```python
from build123d import *

# Parameters (mm, degrees)
BOSS_EXTRUDE1_DEPTH = 30
SKETCH2_W           = 3
SKETCH2_H           = 22
CUT_EXTRUDE1_DEPTH  = 75.999903187
FILLET2_R           = 10
SKETCH5_R           = 2
CUT_EXTRUDE2_DEPTH  = 0.5
SKETCH8_R           = 1
CUT_EXTRUDE3_DEPTH  = 75.983234646
FILLET3_R           = 1
FILLET4_R           = 0.75


with BuildPart() as part:
    # Sketch1 → Boss-Extrude1 (new body)
    with BuildSketch(Plane(origin=(0, 0, 0), x_dir=(1, 0, 0), z_dir=(0, 1, 0))):
        with BuildLine():
            Line((2.436698586, 0.75), (68.683498586, 0.75))
            Line((68.683498586, 0.75), (68.683498586, -0.75))
            Line((68.683498586, -0.75), (2.436698586, -0.75))
            ThreePointArc((2.436698586, -0.75), (1.980263122, -0.860243479), (1.624465724, -1.166666667))
            ThreePointArc((1.624465724, -1.166666667), (-2, 0), (1.624465724, 1.166666667))
            ThreePointArc((1.624465724, 1.166666667), (1.980263122, 0.860243479), (2.436698586, 0.75))
        make_face()
    extrude(amount=BOSS_EXTRUDE1_DEPTH)

    # Sketch2 → Cut-Extrude1 (cut, through all)
    with BuildSketch(Plane.XY.offset(0.75)):
        with Locations((49.664488586, 15)):
            Rectangle(SKETCH2_W, SKETCH2_H)
    extrude(amount=-CUT_EXTRUDE1_DEPTH, mode=Mode.SUBTRACT)

    # Fillet2
    fillet2_edges = [part.edges().sort_by_distance(p)[0] for p in [
        (68.683498586, 30, 0),
        (68.683498586, 0, 0),
    ]]
    fillet(fillet2_edges, radius=FILLET2_R)

    # Sketch5 → Cut-Extrude2 (cut)
    with BuildSketch(Plane(origin=(0, 0, -0.75), x_dir=(-1, 0, 0), z_dir=(0, 0, -1))):
        with Locations((-58.683498586, 20)):
            Circle(SKETCH5_R)
        with Locations((-58.683498586, 10)):
            Circle(SKETCH5_R)
    extrude(amount=-CUT_EXTRUDE2_DEPTH, mode=Mode.SUBTRACT)

    # Sketch8 → Cut-Extrude3 (cut, through all)
    with BuildSketch(Plane(origin=(0, 0, -0.25), x_dir=(-1, 0, 0), z_dir=(0, 0, -1))):
        with Locations((-58.683498586, 20)):
            Circle(SKETCH8_R)
        with Locations((-58.683498586, 10)):
            Circle(SKETCH8_R)
    extrude(amount=-CUT_EXTRUDE3_DEPTH, mode=Mode.SUBTRACT)

    # Fillet3
    fillet3_edges = [part.edges().sort_by_distance(p)[0] for p in [
        (51.164488586, 26, 0),
        (51.164488586, 4, 0),
        (48.164488586, 4, 0),
        (48.164488586, 26, 0),
    ]]
    fillet(fillet3_edges, radius=FILLET3_R)

    # Fillet4
    fillet4_edges = [part.edges().sort_by_distance(p)[0] for p in [
        (48.457381805, 25.707106781, 0.75),
        (49.664488586, 26, 0.75),
        (50.871595367, 25.707106781, 0.75),
        (51.164488586, 15, 0.75),
        (50.871595367, 4.292893219, 0.75),
        (49.664488586, 4, 0.75),
        (48.457381805, 4.292893219, 0.75),
        (48.457381805, 25.707106781, -0.75),
        (49.664488586, 26, -0.75),
        (50.871595367, 25.707106781, -0.75),
        (51.164488586, 15, -0.75),
        (50.871595367, 4.292893219, -0.75),
        (49.664488586, 4, -0.75),
        (48.457381805, 4.292893219, -0.75),
        (48.164488586, 15, 0.75),
        (48.164488586, 15, -0.75),
    ]]
    fillet(fillet4_edges, radius=FILLET4_R - 0.0001)  # a hair under: the kernel refuses the full size


solid = part.part
```
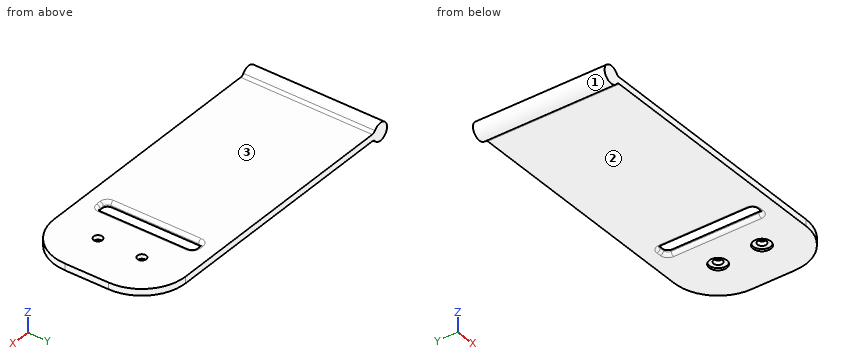
Could you check a few things on this model? Use its own coordinates, in mm. Face numbers are marked on the shaded views. A direction names the side the tool comes from. Round coordinates to 2 decimals unless told otherwise and drop trailing zeros. Loops run counter-clockwise (first coordinate to the right, second up) from the corner with the lowest first, then second, coordinate; pieces in that order, holes last. Notation, with made-up numbers: (5, 63.25) - (59, 63.25) arc R32 cw to (59, 96.25) - close; hole circle Ø3 at (-3, -33.5). An arc over 180 degrees is marked (long way). Answer in a Markdown table with one row per item. Add a question column.
(1) I'm going to push flat-ended pins straight in: pin 1 (9 mm diameter, centred on x = 50, y = 17.5, fed in from -Z); pin 2 (6 mm diameter, centred on x = 23, y = 7.5, fed in from +Z); pin 3 (2.5 mm diameter, centred on x = 58.68, y = 10, fed in from -Z). Where does each tip first touch, or does it pass through?
(2) I need wall thicknesses on line 1 along Z through (x, y) = (47.5, 15.25); line 2 along X through (y, z) = (9.75, -0.4). Which ranges of each line are inside material? Lowest first, please.
(3) If we section it at B-B (x = 54): Please give me the cut outline in (y, z).
(4) For the marked faces 1, 2 and 3, which set-ups out of +Z, -Z, +X, -X, +Y, -Y let a thin tool reach every point of the face, with its end or its side?
(5) If we section it at C-C (x = 64.5): Please give me the cut outline in (y, z), plus the area to 3 significant figures.
Model answer:
| question | item | result |
|---|---|---|
| 1 | pin 1 | stops at z = -0.75 |
| 1 | pin 2 | stops at z = 0.75 |
| 1 | pin 3 | stops at z = -0.25 |
| 2 | line 1 | z = -0.75 to 0.75 |
| 2 | line 2 | x = -1.96 to 48.05, 51.28 to 56.7, 60.67 to 68.68 |
| 3 | outline | (0, -0.75) - (30, -0.75) - (30, 0.75) - (0, 0.75) - close |
| 4 | face 1 | +Y, -Y |
| 4 | face 2 | -Z, +X, +Y, -Y |
| 4 | face 3 | +Z, +X, +Y, -Y |
| 5 | outline | (1.87, -0.75) - (28.13, -0.75) - (28.13, 0.75) - (1.87, 0.75) - close |
| 5 | area | 39.4 mm² |
